Part model, mm, in its own coordinate system. Face numbers are marked on the shaded views. A direction names the side the tool comes from. Give positions to 0.01 mm unless a question says otherwise; leave off trailing zeros. Order: outer loops, then holes, each group sorted by start corner. A loop starts at its lowest first (then second) coordinate and runs counter-clockwise, first axis right, second up. Notation, with made-up numbers: (-37, 23.5) - (0, 23.5) arc R14 cw to (0, 38.5) - close; hole circle Ø8 at (-29, -18.75). An arc over 180 degrees is marked (long way). One line per item, written item: value.
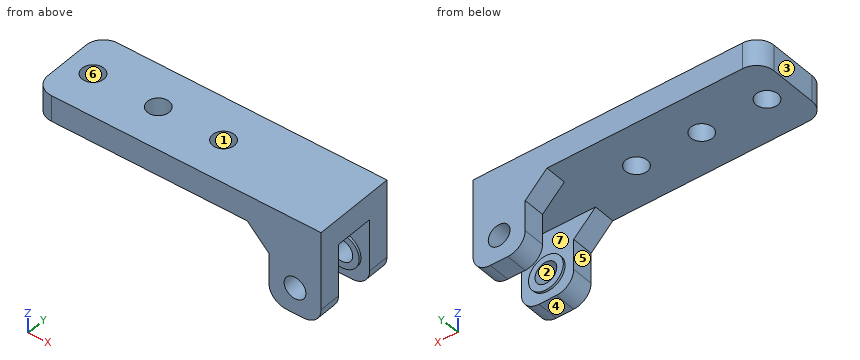
```python
from build123d import *

# Parameters (mm, degrees)
EXTRUDE_1_DEPTH     = 12
SKETCH_2_R          = 2.5
CUT_EXTRUDE_1_DEPTH = 32.448370387
SKETCH_3_R          = 4
SKETCH_3_R_2        = 2.5
EXTRUDE_2_DEPTH     = 0.5
EXTRUDE_START       = 0.5
SKETCH_4_R          = 4
SKETCH_4_R_2        = 2.5
EXTRUDE_3_DEPTH     = 0.5
FILLET_1_R          = 4
EXTRUDE_START_2     = -6
SKETCH_5_W          = 54
SKETCH_5_H          = 19
EXTRUDE_4_DEPTH     = 6
CHAMFER_1_SIZE      = 5
SKETCH_6_R          = 2.5
CUT_EXTRUDE_2_DEPTH = 60.439044407
FILLET_2_R          = 4


with BuildPart() as part:
    # Эскиз1 → Бобышка-Вытянуть1 (new body)
    with BuildSketch(Plane(origin=(0, 0, 0), x_dir=(0, 0, -1), z_dir=(1, 0, 0))):
        Polygon((0, 0), (22, 0), (22, 5), (6, 5), (6, 14), (22, 14), (22, 19), (0, 19), align=None)
    extrude(amount=EXTRUDE_1_DEPTH)

    # Эскиз2 → Вырез-Вытянуть1 (cut, through all)
    with BuildSketch(Plane(origin=(0, 19, 0), x_dir=(1, 0, 0), z_dir=(0, 1, 0))):
        with Locations(Location((6, 16, 0), (0, 0, 270))):
            Circle(SKETCH_2_R)
    extrude(amount=-CUT_EXTRUDE_1_DEPTH, mode=Mode.SUBTRACT)

    # Эскиз3 → Бобышка-Вытянуть2 (add)
    with BuildSketch(Plane.XZ.offset(-14)):
        with Locations(Location((6, -16, 0), (0, 0, 90))):
            Circle(SKETCH_3_R)
        with Locations(Location((6, -16, 0), (0, 0, 90))):
            Circle(SKETCH_3_R_2, mode=Mode.SUBTRACT)
    extrude(amount=EXTRUDE_2_DEPTH)

    # Эскиз4 → Бобышка-Вытянуть3 (add)
    with BuildSketch(Plane(origin=(0, 5, 0), x_dir=(1, 0, 0), z_dir=(0, 1, 0)).offset(EXTRUDE_START)):
        with Locations(Location((6, 16, 0), (0, 0, 270))):
            Circle(SKETCH_4_R)
        with Locations(Location((6, 16, 0), (0, 0, 270))):
            Circle(SKETCH_4_R_2, mode=Mode.SUBTRACT)
    extrude(amount=-EXTRUDE_3_DEPTH)

    # Скругление1
    fillet_1_edges = [part.edges().sort_by_distance(p)[0] for p in [
        (12, 2.5, -22),
        (12, 16.5, -22),
        (0, 16.5, -22),
        (0, 2.5, -22),
    ]]
    fillet(fillet_1_edges, radius=FILLET_1_R)

    # Эскиз5 → Бобышка-Вытянуть4 (add)
    with BuildSketch(Plane.XY.offset(EXTRUDE_START_2)):
        with Locations((-27, 9.5)):
            Rectangle(SKETCH_5_W, SKETCH_5_H)
    extrude(amount=EXTRUDE_4_DEPTH)

    # Фаска1
    chamfer_1_edges = [part.edges().sort_by_distance(p)[0] for p in [
        (0, 16.5, -6),
        (0, 2.5, -6),
    ]]
    chamfer(chamfer_1_edges, length=CHAMFER_1_SIZE)

    # Эскиз6 → Вырез-Вытянуть2 (cut, through all)
    with BuildSketch(Plane(origin=(0, 0, -6), x_dir=(-1, 0, 0), z_dir=(0, 0, -1))):
        with Locations((48, 9.5)):
            Circle(SKETCH_6_R)
        with Locations((33, 9.5)):
            Circle(SKETCH_6_R)
        with Locations((18, 9.5)):
            Circle(SKETCH_6_R)
    extrude(amount=-CUT_EXTRUDE_2_DEPTH, mode=Mode.SUBTRACT)

    # Скругление2
    fillet_2_edges = [part.edges().sort_by_distance(p)[0] for p in [
        (-54, 0, -3),
        (-54, 19, -3),
    ]]
    fillet(fillet_2_edges, radius=FILLET_2_R)


solid = part.part
```
1) Two-plate mould, pull along X, no slides. Class the marked faces 1, 2, 3 and 4: pulls with the +X half, pulls with the -X half, needs draft (parallel to the pull), parting line crosses it, or undercut.
Answer:
face 1: undercut
face 2: undercut
face 3: pulls with the -X half
face 4: needs draft
2) Slice it at A-A on z = -9.75. Write the cut outline in (x, y).
Answer:
outline: (-1.25, 0) - (12, 0) - (12, 5) - (-1.25, 5) - close; (-1.25, 14) - (12, 14) - (12, 19) - (-1.25, 19) - close
3) Wall check: line 1 along Y through (x, z) = (-18, -3.3); line 2 along Z through (x, y) = (6, 16.8); line 3 along Y through (x, z) = (5, -18.5). Give the ranges that are in metal, low to high. Write a range as [from, to].
Answer:
line 1: y = [0, 7], [12, 19]
line 2: z = [-22, -18.5], [-13.5, 0]
line 3: y = [0, 5.5], [13.5, 19]
4) Slice it at B-B on x = -18. Write the cut outline in (y, z), then the cut area to 3 significant figures.
Answer:
outline: (0, -6) - (7, -6) - (7, 0) - (0, 0) - close; (12, -6) - (19, -6) - (19, 0) - (12, 0) - close
area: 84.0 mm2
5) Slice it at D-D on x = 6. Write the cut outline in (y, z), then the cut area to 3 significant figures.
Answer:
outline: (0, -22) - (5, -22) - (5, -20) - (5.5, -20) - (5.5, -18.5) - (0, -18.5) - close; (0, -13.5) - (5.5, -13.5) - (5.5, -12) - (5, -12) - (5, -6) - (14, -6) - (14, -12) - (13.5, -12) - (13.5, -13.5) - (19, -13.5) - (19, 0) - (0, 0) - close; (13.5, -20) - (14, -20) - (14, -22) - (19, -22) - (19, -18.5) - (13.5, -18.5) - close
area: 227 mm2
6) Which spindle directions (+Z, -Z, +X, -X, +Y, -Y) get a long thin tool onto all of the face, cutting with end or side? Do the marked faces 5, 6 and 7. Say none if no direction does.
Answer:
face 5: -Z, -X, +Y, -Y
face 6: +Z, -Z
face 7: none
7) Slice it at C-C on y = 9.5. Write the cut outline in (x, z).
Answer:
outline: (-54, -6) - (-50.5, -6) - (-50.5, 0) - (-54, 0) - close; (-45.5, -6) - (-35.5, -6) - (-35.5, 0) - (-45.5, 0) - close; (-30.5, -6) - (-20.5, -6) - (-20.5, 0) - (-30.5, 0) - close; (-15.5, -6) - (12, -6) - (12, 0) - (-15.5, 0) - close
8) Drop flat-ended pins along their axis: P1, Ø4, axis at y = 3, z = -14, coming from the -X side; P2, Ø8, axis at x = -43.5, y = 10.5, coming from the -Z side; P3, Ø3, axis at y = 4, z = -8, coming from the -X side; P4, Ø4, axis at x = -33, y = 9.5, coming from the -Z side. Give the stop position or say it passes through.
Answer:
P1: stops at x = 0
P2: stops at z = -6
P3: stops at x = -4.5
P4: passes through
